```python
from build123d import *

# Parameters (mm, degrees)
SKETCH1_W           = 30
SKETCH1_H           = 50
BOSS_EXTRUDE1_DEPTH = 1
BOSS_EXTRUDE2_DEPTH = 30
BOSS_EXTRUDE3_DEPTH = 30
BOSS_EXTRUDE5_DEPTH = 30
SKETCH8_W           = 4
SKETCH8_H           = 3.954682566
BOSS_EXTRUDE6_DEPTH = 1


with BuildPart() as part:
    # Sketch1 → Boss-Extrude1 (new body)
    with BuildSketch(Plane(origin=(0, 0, 0), x_dir=(1, 0, 0), z_dir=(0, 1, 0))):
        with Locations((15, 25)):
            Rectangle(SKETCH1_W, SKETCH1_H)
    extrude(amount=BOSS_EXTRUDE1_DEPTH)

    # Sketch3 → Boss-Extrude2 (add)
    with BuildSketch(Plane.ZY):
        with BuildLine():
            Line((-50, 1), (-48, 1))
            ThreePointArc((-48, 1), (-49, 2), (-50, 1))
        make_face()
    boss_extrude2 = extrude(amount=-BOSS_EXTRUDE2_DEPTH)

    # Sketch5 → Boss-Extrude3 (add)
    with BuildSketch(Plane.ZY):
        with BuildLine():
            Line((-46.960567447, 1), (-44.946165632, 1))
            ThreePointArc((-44.946165632, 1), (-45.953366539, 2.007200908), (-46.960567447, 1))
        make_face()
    boss_extrude3 = extrude(amount=-BOSS_EXTRUDE3_DEPTH)

    # Sketch7 → Boss-Extrude5 (add)
    with BuildSketch(Plane.ZY):
        with BuildLine():
            Line((-43.851141388, 1), (-41.851141388, 1))
            ThreePointArc((-41.851141388, 1), (-42.851141388, 2), (-43.851141388, 1))
        make_face()
    boss_extrude5 = extrude(amount=-BOSS_EXTRUDE5_DEPTH)

    # Mirror1: Boss-Extrude2, Boss-Extrude3, Boss-Extrude5 across plane
    add(boss_extrude2.mirror(Plane(origin=(0, 0, -41.5), x_dir=(1, 0, 0), z_dir=(0, 0, -1))))
    add(boss_extrude3.mirror(Plane(origin=(0, 0, -41.5), x_dir=(1, 0, 0), z_dir=(0, 0, -1))))
    add(boss_extrude5.mirror(Plane(origin=(0, 0, -41.5), x_dir=(1, 0, 0), z_dir=(0, 0, -1))))

    # Sketch8 → Boss-Extrude6 (add)
    with BuildSketch(Plane(origin=(0, 1, 0), x_dir=(1, 0, 0), z_dir=(0, 1, 0))):
        with Locations((15, 17.453820001)):
            Rectangle(SKETCH8_W, SKETCH8_H)
    extrude(amount=BOSS_EXTRUDE6_DEPTH)


solid = part.part
```
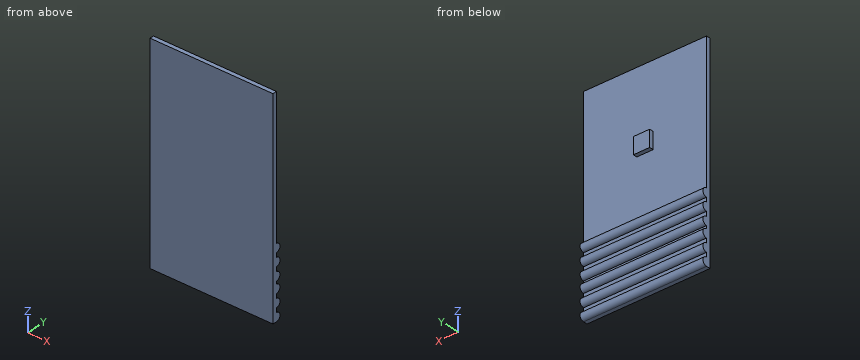
Can you work these out from the model? Positions are in its coordinate system, mm. Coordinates: 2 decimals unless noted, no trailing zeros. Loops run counter-clockwise (first coordinate to the right, second up) from the corner with the lowest first, then second, coordinate; pieces in that order, holes last.
1) Imagine slicing it at C-C on x = 14. List the corners of the cut face in (y, z) for me, plus the area to 3 significant figures.
2) Imagine slicing it at A-A on x = 24.75. List the corners of the cut face in (y, z) for me, plus the area to 3 significant figures.
3) For pin 1 (15 mm diameter, centred on x = 19, z = -13, fed in from +Y); pin 2 (0.5 mm diameter, centred on x = 16, z = -38.5, fed in from +Y); pin 3 (0.5 mm diameter, centred on x = 16, y = 1.5, fed in from -Z), each with a flat end and sliding along its axis, tell me the tip position at first contact or that it passes through.
4) Imagine slicing it at B-B on z = -18. List the corners of the cut face in (x, y) for me.
5) I need wall thicknesses on probe 1 along Z at (x, y) = (27.75, 1.1); probe 2 along Z at (x, y) = (1.75, 1.3); probe 3 along Y at (x, z) = (27.5, -22.5). Which ranges of each line are inside material? Lowest first, please.
6) Imagine slicing it at D-D on z = -6. List the corners of the cut face in (x, y) for me, plus the area to 3 significant figures.
Completed:
1. outline: (0, -50) - (1, -50) arc R1 ccw to (1, -48) - (1, -46.96) arc R1.01 ccw to (1, -44.95) - (1, -43.85) arc R1 ccw to (1, -41.85) - (1, -41.15) arc R1 ccw to (1, -39.15) - (1, -38.05) arc R1.01 ccw to (1, -36.04) - (1, -35) arc R1 ccw to (1, -33) - (1, -19.43) - (2, -19.43) - (2, -15.48) - (1, -15.48) - (1, 0) - (0, 0) - close
1. area: 63.4 mm2
2. outline: (0, -50) - (1, -50) arc R1 ccw to (1, -48) - (1, -46.96) arc R1.01 ccw to (1, -44.95) - (1, -43.85) arc R1 ccw to (1, -41.85) - (1, -41.15) arc R1 ccw to (1, -39.15) - (1, -38.05) arc R1.01 ccw to (1, -36.04) - (1, -35) arc R1 ccw to (1, -33) - (1, 0) - (0, 0) - close
2. area: 59.5 mm2
3. pin 1: stops at y = 2
3. pin 2: stops at y = 1
3. pin 3: stops at z = -49.97
4. outline: (0, 0) - (30, 0) - (30, 1) - (17, 1) - (17, 2) - (13, 2) - (13, 1) - (0, 1) - close
5. probe 1: z = -49.99 to -48.01, -46.96 to -44.95, -43.85 to -41.86, -41.14 to -39.15, -38.05 to -36.04, -34.99 to -33.01
5. probe 2: z = -49.95 to -48.05, -46.91 to -44.99, -43.81 to -41.9, -41.1 to -39.19, -38.01 to -36.09, -34.95 to -33.05
5. probe 3: y = 0 to 1
6. outline: (0, 0) - (30, 0) - (30, 1) - (0, 1) - close
6. area: 30.0 mm2
